```python
from build123d import *

# Parameters (mm, degrees)
SKETCH1_W           = 10
SKETCH1_H           = 10
SKETCH1_R           = 2.605
BOSS_EXTRUDE1_DEPTH = 165.1
CIRPATTERN1_COUNT   = 4
SKETCH2_R           = 2.38
CUT_EXTRUDE6_DEPTH  = 8


with BuildPart() as part:
    # Sketch1 → Boss-Extrude1 (new body)
    with BuildSketch(Plane(origin=(0, 0, 0), x_dir=(0, 0, -1), z_dir=(1, 0, 0))):
        Rectangle(SKETCH1_W, SKETCH1_H)
        Circle(SKETCH1_R, mode=Mode.SUBTRACT)
        Polygon((7.474873734, 9.921463197), (2.553410537, 5), (5, 5), (5, 3.203948776), (9.596194078, 7.800142853), align=None)
        Polygon((9.596194078, 3.24), (12.596194078, 3.24), (12.596194078, 12.596194078), (3.24, 12.596194078), (3.24, 9.921463197), (7.474873734, 9.921463197), (9.596194078, 7.800142853), align=None)
    boss_extrude1 = extrude(amount=BOSS_EXTRUDE1_DEPTH)

    # CirPattern1: Boss-Extrude1 ×4 about axis
    cirpattern1_axis = Axis((0, 0, 0), (1, 0, 0))
    for i in range(1, CIRPATTERN1_COUNT):
        add(boss_extrude1.rotate(cirpattern1_axis, i * 360 / CIRPATTERN1_COUNT))

    # Sketch2 → Cut-Extrude6 (cut)
    with BuildSketch(Plane.XY.offset(12.596194078)):
        with Locations((86.36, 0)):
            Circle(SKETCH2_R)
    extrude(amount=-CUT_EXTRUDE6_DEPTH, mode=Mode.SUBTRACT)


solid = part.part
```
Can you work these out from the model? Positions are in its coordinate system, mm. A direction names the side the tool comes from. Coordinates: 2 decimals unless noted, no trailing zeros. Order: outer loops, then holes, each group sorted by start corner. A loop starts at its lowest first (then second) coordinate and runs counter-clockwise, first axis right, second up. Notation, with made-up numbers: (19, 5) - (67, 5) arc R21 ccw to (67, 25) - close; hole circle Ø11 at (19.25, 75). An arc over 180 degrees is marked (long way). Answer in a Markdown table with one row per item.
1. If I drill on line 1 along Z through (x, y) = (156.5, -6.5); line 2 along Y through (x, z) = (59, -6.5); line 3 along Y through (x, z) = (62, 6.75), over which ranges is the centre line in solid material (lowest first)?
Reply:
| item | result |
|---|---|
| line 1 | z = -12.6 to -9.92, -8.95 to -4.7, 4.05 to 8.3, 9.6 to 12.6 |
| line 2 | y = -12.6 to -9.6, -8.3 to -4.05, 4.7 to 8.95, 9.92 to 12.6 |
| line 3 | y = -12.6 to -9.92, -9.2 to -4.95, 4.3 to 8.55, 9.6 to 12.6 |
2. Suppose I cut it at A-A (y = 0). Please give me the cut outline in (x, z) (3 decimals).
Reply:
| item | result |
|---|---|
| outline | (0, -5) - (165.1, -5) - (165.1, -2.605) - (0, -2.605) - close; (0, 2.605) - (165.1, 2.605) - (165.1, 5) - (88.74, 5) - (88.74, 4.596) - (83.98, 4.596) - (83.98, 5) - (0, 5) - close |
3. For faces 1 (the flat face through (81, -5, 0)), 2 (the flat face through (81, 11, 3.24)), 3 (the flat face through (81, 8, 12.596)), which set-ups out of +Z, -Z, +X, -X, +Y, -Y let a thin tool reach every point of the face, with its end or its side?
Reply:
| item | result |
|---|---|
| face 1 | +X, -X, -Y |
| face 2 | +X, -X, +Y |
| face 3 | +Z, +X, -X, +Y, -Y |
4. For pin 1 (1.7 mm diameter, centred on x = 73, y = 0.5, fed in from +Z), with a flat end and sliding along its axis, tell me the tip position at first contact or that it passes through.
Reply:
| item | result |
|---|---|
| pin 1 | stops at z = 5 |
5. If we mould it in two halves opening along Z, with no side actions, what happens to faces 4 (the flat face through (81, -3.24, -11)), 5 (the flat face through (81, 5, 0)), 6 (the flat face through (81, -8, 12.596)), 7 (the flat face through (81, 0, -5))? For each: pulls with the +Z half, pulls with the -Z half, needs draft (parallel to the pull), parting line crosses it, or undercut.
Reply:
| item | result |
|---|---|
| face 4 | needs draft |
| face 5 | undercut |
| face 6 | pulls with the +Z half |
| face 7 | pulls with the -Z half |
